from build123d import *

# Parameters (mm, degrees)
SKETCH_1_R          = 1.205
EXTRUDE_1_DEPTH     = 3.175
SKETCH_2_W          = 0.5
SKETCH_2_H          = 3.63
EXTRUDE_2_DEPTH     = 3.08
SKETCH_3_R          = 0.735
CUT_EXTRUDE_1_DEPTH = 21.998730652
SKETCH_4_W          = 6.4
SKETCH_4_H          = 3.75
CUT_EXTRUDE_2_DEPTH = 1
SKETCH_6_W          = 21.6
SKETCH_6_H          = 3.75
EXTRUDE_3_DEPTH     = 0.5


with BuildPart() as part:
    # 스케치1 → 보스-돌출1 (new, symmetric)
    with BuildSketch(Plane.XY):
        Polygon((-14.02, -2.36), (5.82, -2.36), (5.82, 6.58), (-4.42, 6.58), (-5.01, 7.17), (-7.62, 7.17), (-7.62, 9.908), (-14.02, 9.908), (-14.02, 6.58), align=None)
        Circle(SKETCH_1_R, mode=Mode.SUBTRACT)
        with BuildLine():
            Line((-10.212788401, 1.205), (-8.847211599, 1.205))
            ThreePointArc((-8.847211599, 1.205), (-8.145, 0), (-8.847211599, -1.205))
            Line((-8.847211599, -1.205), (-10.212788401, -1.205))
            ThreePointArc((-10.212788401, -1.205), (-10.915, 0), (-10.212788401, 1.205))
        make_face(mode=Mode.SUBTRACT)
    extrude(amount=EXTRUDE_1_DEPTH, both=True)

    # 스케치2 → 보스-돌출2 (add)
    with BuildSketch(Plane.XZ.offset(2.36)):
        with Locations((-12.17, 0)):
            Rectangle(SKETCH_2_W, SKETCH_2_H)
        with Locations((-1.88, 0)):
            Rectangle(SKETCH_2_W, SKETCH_2_H)
        with Locations((4.14, 0)):
            Rectangle(SKETCH_2_W, SKETCH_2_H)
    extrude(amount=EXTRUDE_2_DEPTH)

    # 스케치3 → 컷-돌출1 (cut, through all)
    with BuildSketch(Plane.ZY.offset(12.42)):
        with Locations(Location((0, -3.9, 0), (0, 0, 270))):
            Circle(SKETCH_3_R)
    extrude(amount=-CUT_EXTRUDE_1_DEPTH, mode=Mode.SUBTRACT)

    # 스케치4 → 컷-돌출2 (cut)
    with BuildSketch(Plane(origin=(0, 9.908, 0), x_dir=(1, 0, 0), z_dir=(0, 1, 0))):
        with Locations((-10.82, 0)):
            Rectangle(SKETCH_4_W, SKETCH_4_H)
    extrude(amount=-CUT_EXTRUDE_2_DEPTH, mode=Mode.SUBTRACT)

    # 스케치6 → 보스-돌출3 (add)
    with BuildSketch(Plane(origin=(0, 8.908, 0), x_dir=(1, 0, 0), z_dir=(0, 1, 0))):
        with Locations((-3.22, 0)):
            Rectangle(SKETCH_6_W, SKETCH_6_H)
    extrude(amount=-EXTRUDE_3_DEPTH)


solid = part.part
The listing builds one solid part. Answer for the finished solid, in the listing's coordinates (mm). A direction names the side the tool comes from. Coordinates: 2 decimals unless noted, no trailing zeros. Loops run counter-clockwise (first coordinate to the right, second up) from the corner with the lowest first, then second, coordinate; pieces in that order, holes last. Notation, with made-up numbers: (-6, 37) -> (3, 37) arc R30 cw to (3, 73) -> close; hole circle Ø4 at (-34.75, 40.5). An arc over 180 degrees is marked (long way). Write item = value, one per line. Start each with the question number.
1) The mould has two halves that part along Y. Classify faces 1 (the face through (-6, 7.17, 0)), 2 (the face through (-3, 8.908, 0)), 3 (the face through (4.39, -3, 0)): released by +Y, released by -Y, zero draft, split by the parting line, or undercut.
2) Given pin 1 Ø1.5 at (y, z) = (-4.5, -1) entering from +X; pin 2 Ø0.6 at (x, y) = (4, -3.5) entering from +Z (3 decimals); pin 3 Ø1 at (x, z) = (-3, 0) entering from +Y, each flat-ended and moving along its own axis, determine where each tip first touches the part or whether it passes through.
3) Straight lines are drawn through the part: line 1 (X direction, y = -3, z = 0.25); line 2 (Y direction, x = -2.5, z = 1.75); line 3 (X direction, y = -0.25, z = -2.5). For each, find the intervals that lie inside material, in ascending order. Write a range as from..to.
4) A cutting plane is placed at B-B (y = 0). Give the vertices of the cut face in (x, z) (3 decimals).
5) A cutting plane is placed at A-A (x = 0). Give the vertices of the cut face in (y, z) (3 decimals), then the cut area to 3 significant figures.
6) A cutting plane is placed at C-C (z = -1). Give the vertices of the cut face in (x, y) (3 decimals), then the cut area to 3 significant figures.
7) A cutting plane is placed at D-D (y = -3.9). Give the vertices of the cut face in (x, z) (3 decimals), then the cut area to 3 significant figures.
8) A tool of negligible diameter and unlimited length cuts with its end or side. For faces 4 (the face through (-1.63, -3, 0)), 5 (the face through (-12.42, -3, 0)), 6 (the face through (-10.915, -0.02, 0.044)), 7 (the face through (-10.9, 9.4, 1.875)), from which of +Z, -Z, +X, -X, +Y, -Y can it reach the whole face along a straight path? Write none if from no direction.
Responses:
q1.face_1 = undercut
q1.face_2 = released by +Y
q1.face_3 = zero draft
q2.pin_1 = 4.39
q2.pin_2 = 1.815
q2.pin_3 = 8.91
q3.line_1 = -12.42..-11.92, -2.13..-1.63, 3.89..4.39
q3.line_2 = -2.36..6.58, 8.41..8.91
q3.line_3 = -14.02..-10.89, -8.17..-1.18, 1.18..5.82
q4.outline = (-14.02, -3.175) -> (-10.915, -3.175) -> (-10.915, 3.175) -> (-14.02, 3.175) -> close; (-8.145, -3.175) -> (-1.205, -3.175) -> (-1.205, 3.175) -> (-8.145, 3.175) -> close; (1.205, -3.175) -> (5.82, -3.175) -> (5.82, 3.175) -> (1.205, 3.175) -> close
q5.outline = (-2.36, -3.175) -> (-1.205, -3.175) -> (-1.205, 3.175) -> (-2.36, 3.175) -> close; (1.205, -3.175) -> (6.58, -3.175) -> (6.58, 3.175) -> (1.205, 3.175) -> close; (8.408, -1.875) -> (8.908, -1.875) -> (8.908, 1.875) -> (8.408, 1.875) -> close
q5.area = 43.3 mm²
q6.outline = (-14.02, -2.36) -> (-12.42, -2.36) -> (-12.42, -5.44) -> (-11.92, -5.44) -> (-11.92, -2.36) -> (-2.13, -2.36) -> (-2.13, -5.44) -> (-1.63, -5.44) -> (-1.63, -2.36) -> (3.89, -2.36) -> (3.89, -5.44) -> (4.39, -5.44) -> (4.39, -2.36) -> (5.82, -2.36) -> (5.82, 6.58) -> (-4.42, 6.58) -> (-5.01, 7.17) -> (-7.62, 7.17) -> (-7.62, 8.408) -> (7.58, 8.408) -> (7.58, 8.908) -> (-14.02, 8.908) -> close; hole (-10.213, -1.205) -> (-8.847, -1.205) arc R1.385 ccw to (-8.847, 1.205) -> (-10.213, 1.205) arc R1.385 ccw to start; hole circle Ø2.41 at (0, 0)
q6.area = 196 mm²
q7.outline = (-12.42, -1.815) -> (-11.92, -1.815) -> (-11.92, -0.735) -> (-12.42, -0.735) -> close; (-12.42, 0.735) -> (-11.92, 0.735) -> (-11.92, 1.815) -> (-12.42, 1.815) -> close; (-2.13, -1.815) -> (-1.63, -1.815) -> (-1.63, -0.735) -> (-2.13, -0.735) -> close; (-2.13, 0.735) -> (-1.63, 0.735) -> (-1.63, 1.815) -> (-2.13, 1.815) -> close; (3.89, -1.815) -> (4.39, -1.815) -> (4.39, -0.735) -> (3.89, -0.735) -> close; (3.89, 0.735) -> (4.39, 0.735) -> (4.39, 1.815) -> (3.89, 1.815) -> close
q7.area = 3.24 mm²
q8.face_4 = +Z, -Z, -Y
q8.face_5 = +Z, -Z, -X, -Y
q8.face_6 = +Z, -Z
q8.face_7 = +X, -X, +Y
